Here's how the part is built. I have some questions about the finished solid (model axes, mm). A direction names the side the tool comes from. Give positions to 0.01 mm unless a question says otherwise; leave off trailing zeros. Loops run counter-clockwise (first coordinate to the right, second up) from the corner with the lowest first, then second, coordinate; pieces in that order, holes last. Notation, with made-up numbers: (-22.5, -19.75) -> (5.5, -19.75) arc R25 ccw to (5.5, -5.75) -> close; hole circle Ø11 at (58, 53.25). An arc over 180 degrees is marked (long way). Answer in a Markdown table with one row per item. Add a question column.
Item 1: If we section it at A-A (y = -26.5): Write out the boundary of the cut face in (x, z).
Item 2: If we section it at B-B (z = -10): Write out the boundary of the cut face in (x, y), then the cut area to 3 significant figures.
Item 3: Which directions (+Z, -Z, +X, -X, +Y, -Y) give clear straight access to the entire face, cutting with the end or side of a thin tool? Please do faces 1 (the face through (-13, -13.69, -51)), 2 (the face through (-13, -33, -21.6)), 3 (the face through (-13, 3, -18.4)).
Item 4: If we section it at D-D (z = -57): Write out the boundary of the cut face in (x, y), then the cut area to 3 significant figures.
Item 5: We'd pull the mould along Y, two halves only. Please class faces 4 (the face through (-13, -3, -21.6)), 5 (the face through (-13, 5.31, -25)), 6 (the face through (-13, -20.69, -37)): released by +Y, released by -Y, zero draft, split by the parting line, or undercut.
Item 6: For P1, Ø1.3, axis at x = -13, z = -18, coming from the +Y side; P2, Ø1, axis at y = -17, z = -35.5, coming from the +X side; P3, Ø1.5, axis at x = -13, y = -36.5, coming from the -Z side; P4, Ø0.6, axis at x = -14, z = -22, coming from the -Y side, each with a flat end and sliding along its axis, tell me the tip position at first contact or that it passes through.
Item 7: If I drill on line 1 (Y direction, x = -12.8, z = -37); line 2 (Y direction, x = -13.1, z = -57); line 3 (Y direction, x = -13.4, z = -10), over which ranges is the centre line in solid material (lowest first)?
Item 8: If we section it at C-C (z = -37): Write out the boundary of the cut face in (x, y), then the cut area to 3 significant figures.
```python
from build123d import *

# Parameters (mm, degrees)
SKETCH024_W                = 40
SKETCH024_H                = 27
SKETCH024_R                = 1.9
PAD010_DEPTH               = 3
SKETCH025_W                = 3
SKETCH025_H                = 6
PAD011_DEPTH               = 3
SKETCH025_MIRRORED003_2_W  = 3
SKETCH025_MIRRORED003_2_H  = 6
PAD011_MIRRORED003_2_DEPTH = 3
POCKET014_DEPTH            = 109.846683
SKETCH027_R                = 4.5
SKETCH027_W                = 40
SKETCH027_H                = 50
PAD012_DEPTH               = 3
SKETCH028_R                = 1.65
SKETCH028_W                = 12
SKETCH028_H                = 5
POCKET015_DEPTH            = 3.001
SKETCH029_R                = 3.75
SKETCH029_W                = 2
SKETCH029_H                = 2
POCKET016_DEPTH            = 3.001


with BuildPart() as part:
    # Sketch024 → Pad010 (new body)
    with BuildSketch(Plane.YZ):
        Rectangle(SKETCH024_W, SKETCH024_H)
        with Locations((0, 8.5)):
            Circle(SKETCH024_R, mode=Mode.SUBTRACT)
    extrude(amount=PAD010_DEPTH)

    # Sketch025 (on Face7 of Pad010) → Pad011 (join)
    with BuildSketch(Plane.YZ.offset(3)):
        with Locations((-21.5, 10.5)):
            Rectangle(SKETCH025_W, SKETCH025_H)
    pad011 = extrude(amount=-PAD011_DEPTH)

    # Sketch025 Mirrored003 2 → Pad011 Mirrored003 2 (add)
    with BuildSketch(Plane(origin=(3, 0, 0), x_dir=(0, -1, 0), z_dir=(-1, 0, 0))):
        with Locations((-21.5, 10.5)):
            Rectangle(SKETCH025_MIRRORED003_2_W, SKETCH025_MIRRORED003_2_H)
    pad011_mirrored003_2 = extrude(amount=PAD011_MIRRORED003_2_DEPTH)

    # Mirrored005: Pad011, Pad011 Mirrored003 2 across Sketch025 H_Axis
    add(pad011.mirror(Plane(origin=(3, 0, 0), x_dir=(1, 0, 0), z_dir=(0, 0, 1))))
    add(pad011_mirrored003_2.mirror(Plane(origin=(3, 0, 0), x_dir=(1, 0, 0), z_dir=(0, 0, 1))))

    # Sketch026 (on Face12 of MultiTransform001) → Pocket014 (cut, through all)
    with BuildSketch(Plane.YZ.offset(3)):
        Polygon((-20, 1.6), (-16, 1.6), (-16, 2.75), (-13.5, 2.75), (-13.5, 1.6), (-10, 1.6), (-10, -1.6), (-13.5, -1.6), (-13.5, -2.75), (-16, -2.75), (-16, -1.6), (-20, -1.6), align=None)
    pocket014 = extrude(amount=-POCKET014_DEPTH, mode=Mode.SUBTRACT)

    # Mirrored004: Pocket014 across Sketch026 V_Axis
    add(pocket014.mirror(Plane(origin=(3, 0, 0), x_dir=(1, 0, 0), z_dir=(0, 1, 0))), mode=Mode.SUBTRACT)

    # Sketch027 (on Face5 of Mirrored004) → Pad012 (join)
    with BuildSketch(Plane(origin=(0, 0, 0), x_dir=(0, 1, 0), z_dir=(-1, 0, 0))):
        with Locations((0, -8.5)):
            Circle(SKETCH027_R)
        with Locations((0, 32.5)):
            Rectangle(SKETCH027_W, SKETCH027_H)
    extrude(amount=-PAD012_DEPTH)

    # Sketch028 (on Face42 of Pad012) → Pocket015 (cut, through all)
    with BuildSketch(Plane(origin=(0, 0, 0), x_dir=(0, 1, 0), z_dir=(-1, 0, 0))):
        with Locations((-15, 17)):
            Circle(SKETCH028_R)
        with Locations((15, 17)):
            Circle(SKETCH028_R)
        with Locations((15, -10)):
            Circle(SKETCH028_R)
        with Locations((-15, -10)):
            Circle(SKETCH028_R)
        with Locations((0, 17)):
            Rectangle(SKETCH028_W, SKETCH028_H)
    extrude(amount=-POCKET015_DEPTH, mode=Mode.SUBTRACT)

    # Sketch029 (on Face2 of Pocket015) → Pocket016 (cut, through all)
    with BuildSketch(Plane(origin=(0, 0, 0), x_dir=(0, 1, 0), z_dir=(-1, 0, 0))):
        with Locations((0, 37)):
            Circle(SKETCH029_R)
        with Locations((0, 31)):
            Rectangle(SKETCH029_W, SKETCH029_H)
    extrude(amount=-POCKET016_DEPTH, mode=Mode.SUBTRACT)


with BuildPart() as part_1:
    # Body006 placement: moved
    add(part.part.moved(Location((-14.7217, -14.6897, -20))))


solid = part_1.part
```
Recorded:
| question | item | result |
|---|---|---|
| 1 | outline | (-14.72, -77.5) -> (-11.72, -77.5) -> (-11.72, -21.6) -> (-14.72, -21.6) -> close; (-14.72, -18.4) -> (-11.72, -18.4) -> (-11.72, -6.5) -> (-14.72, -6.5) -> close |
| 2 | outline | (-14.72, -37.69) -> (-11.72, -37.69) -> (-11.72, -31.34) -> (-14.72, -31.34) -> close; (-14.72, -28.04) -> (-11.72, -28.04) -> (-11.72, -1.34) -> (-14.72, -1.34) -> close; (-14.72, 1.96) -> (-11.72, 1.96) -> (-11.72, 8.31) -> (-14.72, 8.31) -> close |
| 2 | area | 118 mm^2 |
| 3 | face 1 | +X, -X |
| 3 | face 2 | +X, -X, -Y |
| 3 | face 3 | +X, -X, +Y |
| 4 | outline | (-14.72, -34.69) -> (-11.72, -34.69) -> (-11.72, -18.44) -> (-14.72, -18.44) -> close; (-14.72, -10.94) -> (-11.72, -10.94) -> (-11.72, 5.31) -> (-14.72, 5.31) -> close |
| 4 | area | 97.5 mm^2 |
| 5 | face 4 | zero draft |
| 5 | face 5 | released by +Y |
| 5 | face 6 | undercut |
| 6 | P1 | stops at y = 5.31 |
| 6 | P2 | passes through |
| 6 | P3 | stops at z = -33.5 |
| 6 | P4 | stops at y = -34.69 |
| 7 | line 1 | y = -34.69 to -31.34, -28.04 to -20.69, -8.69 to -1.34, 1.96 to 5.31 |
| 7 | line 2 | y = -34.69 to -18.44, -10.94 to 5.31 |
| 7 | line 3 | y = -37.69 to -31.34, -28.04 to -1.34, 1.96 to 8.31 |
| 8 | outline | (-14.72, -34.69) -> (-11.72, -34.69) -> (-11.72, -31.34) -> (-14.72, -31.34) -> close; (-14.72, -28.04) -> (-11.72, -28.04) -> (-11.72, -20.69) -> (-14.72, -20.69) -> close; (-14.72, -8.69) -> (-11.72, -8.69) -> (-11.72, -1.34) -> (-14.72, -1.34) -> close; (-14.72, 1.96) -> (-11.72, 1.96) -> (-11.72, 5.31) -> (-14.72, 5.31) -> close |
| 8 | area | 64.2 mm^2 |
